Part model, mm, in its own coordinate system. A direction names the side the tool comes from. Give positions to 0.01 mm unless a question says otherwise; leave off trailing zeros. Write each loop counter-clockwise with the first axis right and the second up, starting at its lowest first coordinate (ties: lowest second). Pieces come first, ordered by that corner, then holes.
from build123d import *

# Parameters (mm, degrees)
SKETCH5_R   = 6.35
SKETCH5_R_2 = 5.969


with BuildPart() as part:
    # Sweep1: sweep along a path in Sketch4
    with BuildLine(Plane.XY) as sweep1_path:
        Line((121.865926636, 47.432526586), (95.091694349, 47.432526586))
        ThreePointArc((95.091694349, 47.432526586), (72.177912426, 43.905758233), (51.385169899, 33.651912361))
        Line((51.385169899, 33.651912361), (-34.092088176, -26.199908089))
        ThreePointArc((-34.092088176, -26.199908089), (-54.884830704, -36.453753961), (-77.798612626, -39.980522314))
        Line((-77.798612626, -39.980522314), (-104.572844914, -39.980522314))
    # Sketch5 → Sweep1 (sweep)
    with BuildSketch(Plane(origin=(121.865926636, 47.432526586, 0), x_dir=(0, 0, 1), z_dir=(-1, 0, 0))):
        Circle(SKETCH5_R)
        Circle(SKETCH5_R_2, mode=Mode.SUBTRACT)
    sweep(path=sweep1_path.line)


solid = part.part
1) 3-axis set-ups, long thin cutter, end or side, ignore diameter. For faces 1 (the cylindrical face through (108.291, 42.137, 2.754)), 2 (the cylindrical face through (-91.373, -34.626, 3.414)): which of +Z, -Z, +X, -X, +Y, -Y reach the whole face in a straight line?
Check result:
face 1: +X
face 2: -X
2) Saw through at A-A (z = 0). Write the cut outline in (x, y).
Check result:
outline: (-104.57, -46.33) - (-77.8, -46.33) arc R82.55 ccw to (-30.45, -31.4) - (55.03, 28.45) arc R69.85 cw to (95.09, 41.08) - (121.87, 41.08) - (121.87, 41.46) - (95.09, 41.46) arc R70.23 ccw to (54.81, 28.76) - (-30.67, -31.09) arc R82.17 cw to (-77.8, -45.95) - (-104.57, -45.95) - close; (-104.57, -34.01) - (-77.8, -34.01) arc R70.23 ccw to (-37.52, -21.31) - (47.96, 38.54) arc R82.17 cw to (95.09, 53.4) - (121.87, 53.4) - (121.87, 53.78) - (95.09, 53.78) arc R82.55 ccw to (47.74, 38.85) - (-37.73, -21) arc R69.85 cw to (-77.8, -33.63) - (-104.57, -33.63) - close
3) Flat gauge pins, fed straight in: P1, Ø2, axis at x = 65, z = 3.5, coming from the +Y side; P2, Ø5, axis at y = 42, z = 0, coming from the -X side; P3, Ø1, axis at x = 48.5, y = 32.5, coming from the +Z side. Where does each tip first touch, or does it go through?
Check result:
P1: stops at y = 47.69
P2: stops at x = 48.68
P3: stops at z = 6.35
4) Drill centre lines: L1, parallel to Y at x = -93.25, z = 0; L2, parallel to X at y = -12.5, z = -0.75; L3, parallel to Y at x = 41, z = -1.5. Where is each one in solid material? Low to high.
Check result:
L1: y = -46.33 to -45.95, -34.01 to -33.63
L2: x = -25.52 to -24.85, -4.2 to -3.53
L3: y = 18.85 to 19.33, 33.43 to 33.91
5) Mould opens along X. For faces 3 (the cylindrical face through (11.604, -1.771, -1.377)), 4 (the cylindrical face through (-91.37, -45.28, 2.75)), 5 (the flat face through (121.866, 51, -5)), 6 (the cylindrical face through (7.898, 3.522, -5.963)) say: +X half, -X half, draft (parallel to the pull), parting line (faces both ways), or undercut.
Check result:
face 3: parting line
face 4: draft
face 5: +X half
face 6: undercut
